Design review of the part built by this model. Coordinates are the model's own, in mm. A direction names the side the tool comes from. Round coordinates to 2 decimals unless told otherwise and drop trailing zeros. Loops run counter-clockwise (first coordinate to the right, second up) from the corner with the lowest first, then second, coordinate; pieces in that order, holes last. Notation, with made-up numbers: M -4.5,-36 L 42.5,-36 A30 cw 42.5,-13 Z; hole C -19.75,53 d7. An arc over 180 degrees is marked long. Use a Markdown table: item, result.
from build123d import *

# Parameters (mm, degrees)
SKETCH1_W                           = 139.991389113
SKETCH1_H                           = 97.393342316
PICOVER_DEPTH                       = 40
PICOVER_DEPTH_BACK                  = 2
SKETCH2_W                           = 96.759944342
SKETCH2_H                           = 90.25941534
OPENINGFORPI_DEPTH                  = 37
SKETCH3_R                           = 23.23056694
HOLETOACCESSSDCARD_DEPTH            = 7.133927
SKETCH4_W                           = 18
SKETCH4_H                           = 97.393342316
CUTAWAYSTHATDEFINESCREWPLATES_DEPTH = 30
BOSS_EXTRUDE1_DEPTH                 = 97.393342
SKETCH6_W                           = 63.672875613
SKETCH6_H                           = 37
HOLEFORPOWERHDMIAUDIO_DEPTH         = 30
SKETCH5_R                           = 2.75
CUT_EXTRUDE5_DEPTH                  = 43
SKETCH7_R                           = 2.75
CUT_EXTRUDE7_DEPTH                  = 30
FILLET1_R                           = 30
FILLET2_R                           = 30


with BuildPart() as part:
    # Sketch1 → PiCover (new body, two sides)
    with BuildSketch(Plane(origin=(0, 0, 0), x_dir=(1, 0, 0), z_dir=(0, 1, 0))) as picover_sk:
        with Locations((69.995694556, 48.696671158)):
            Rectangle(SKETCH1_W, SKETCH1_H)
    extrude(amount=PICOVER_DEPTH)
    extrude(picover_sk.sketch, amount=-PICOVER_DEPTH_BACK)

    # Sketch2 → OpeningForPi (cut)
    with BuildSketch(Plane(origin=(0, 40, 0), x_dir=(1, 0, 0), z_dir=(0, 1, 0))):
        with Locations((70.044375284, 52.263634646)):
            Rectangle(SKETCH2_W, SKETCH2_H)
    extrude(amount=-OPENINGFORPI_DEPTH, mode=Mode.SUBTRACT)

    # Sketch3 → HoleToAccessSDCard (cut)
    with BuildSketch(Plane.XY):
        with Locations((67.175241294, 40)):
            Circle(SKETCH3_R)
    extrude(amount=-HOLETOACCESSSDCARD_DEPTH, mode=Mode.SUBTRACT)

    # Sketch4 → CutAwaysThatDefineScrewPlates (cut)
    with BuildSketch(Plane.XZ.offset(2)):
        with Locations((130.991389113, -48.696671158)):
            Rectangle(SKETCH4_W, SKETCH4_H)
        with Locations((9, -48.696671158)):
            Rectangle(SKETCH4_W, SKETCH4_H)
    extrude(amount=-CUTAWAYSTHATDEFINESCREWPLATES_DEPTH, mode=Mode.SUBTRACT)

    # Sketch11 → Boss-Extrude1 (add)
    with BuildSketch(Plane.XY):
        Polygon((0, 28), (18, 28), (18, -2), align=None)
        Polygon((139.991389113, 28), (121.991389113, 28), (121.991389113, -2), align=None)
    extrude(amount=-BOSS_EXTRUDE1_DEPTH)

    # Sketch6 → HoleForPowerHDMIAudio (cut)
    with BuildSketch(Plane(origin=(21.664403113, 0, 0), x_dir=(0, 0, -1), z_dir=(1, 0, 0))):
        with Locations((44.503037234, 21.5)):
            Rectangle(SKETCH6_W, SKETCH6_H)
    extrude(amount=-HOLEFORPOWERHDMIAUDIO_DEPTH, mode=Mode.SUBTRACT)

    # Sketch5 → Cut-Extrude5 (cut, through all)
    with BuildSketch(Plane(origin=(0, 40, 0), x_dir=(1, 0, 0), z_dir=(0, 1, 0))):
        with Locations((129.624485255, 49.878598174)):
            Circle(SKETCH5_R)
    extrude(amount=-CUT_EXTRUDE5_DEPTH, mode=Mode.SUBTRACT)

    # Sketch7 → Cut-Extrude7 (cut)
    with BuildSketch(Plane(origin=(0, 40, 0), x_dir=(1, 0, 0), z_dir=(0, 1, 0))):
        with Locations((6.934452889, 8.128892452)):
            Circle(SKETCH7_R)
        with Locations((6.934452889, 91.275593332)):
            Circle(SKETCH7_R)
    extrude(amount=-CUT_EXTRUDE7_DEPTH, mode=Mode.SUBTRACT)

    # Fillet1
    fillet1_edges = [part.edges().sort_by_distance(p)[0] for p in [
        (21.664403113, 3, -86.866408678),
    ]]
    fillet(fillet1_edges, radius=FILLET1_R)

    # Fillet2
    fillet2_edges = [part.edges().sort_by_distance(p)[0] for p in [
        (118.424347455, 3, -52.263634646),
    ]]
    fillet(fillet2_edges, radius=FILLET2_R)


solid = part.part
1. The part is to be moulded in two halves that separate along Z. For faces 1 (the face through (126, 40, -49)), 2 (the face through (126.877, 26.996, -50)), 3 (the face through (71, 15, 0)), say which applies: pulls with the +Z half, pulls with the -Z half, needs draft (parallel to the pull), parting line crosses it, or undercut.
Check values:
| item | result |
|---|---|
| face 1 | needs draft |
| face 2 | undercut |
| face 3 | pulls with the +Z half |
2. Take a section at D-D on x = 25.5. Give the boundary of the cut face in (y, z).
Check values:
| item | result |
|---|---|
| outline | M -2,-97.39 L 18.32,-97.39 L 18.32,-76.34 L 3,-76.34 L 3,-7.13 L 40,-7.13 L 40,0 L -2,0 Z |
3. Take a section at C-C on z = -58. Give the boundary of the cut face in (x, y), and give its area (3 significant figures).
Check values:
| item | result |
|---|---|
| outline | M 15,3 L 18,-2 L 121.99,-2 L 139.99,28 L 139.99,40 L 118.42,40 L 118.42,33 A30 cw 88.42,3 Z |
| area | 1,340 mm² |
4. Insertion check: pin 1 (4.5 mm diameter, centred on y = 24.5, z = -9.5, fed in from +X); pin 2 (3 mm diameter, centred on y = 31.5, z = -45, fed in from -X); pin 3 (9 mm diameter, centred on x = 129.62, z = -49.88, fed in from -Y). Each pin has a flat end and moves straight along its axis. Give the tip position at first contact, or say it passes through.
Check values:
| item | result |
|---|---|
| pin 1 | stops at x = 139.24 |
| pin 2 | stops at x = 118.27 |
| pin 3 | stops at y = 3.21 |
5. Take a section at B-B on y = 35. Give the boundary of the cut face in (x, z).
Check values:
| item | result |
|---|---|
| outline | M 0,-97.39 L 21.66,-97.39 L 21.66,-76.34 L 0,-76.34 Z; M 0,-12.67 L 21.66,-12.67 L 21.66,-7.13 L 44.49,-7.13 L 44.49,0 L 0,0 Z; M 89.86,-7.13 L 118.42,-7.13 L 118.42,-97.39 L 139.99,-97.39 L 139.99,0 L 89.86,0 Z; hole C 6.93,-91.28 d5.5; hole C 6.93,-8.13 d5.5; hole C 129.62,-49.88 d5.5 |
6. Machinability: for faces 4 (the face through (30.69, 11.55, -87.01)), 5 (the face through (13, 25, -12.667)), 6 (the face through (22, 40, -5)), which of the approach directions +Z, -Z, +X, -X, +Y, -Y give a long, thin tool a straight path to every point of the face, cutting with its end or side? Answer none if there is none.
Check values:
| item | result |
|---|---|
| face 4 | -Z, +Y |
| face 5 | -X, +Y |
| face 6 | +Z, -Z, +X, -X, +Y |
7. Wall thickness on line 1 along Z through (x, y) = (6.5, 38.5); line 2 along X through (y, z) = (36, -92.5); line 3 along Z through (x, y) = (116, 36): over which ranges is each line inside the solid? List them lowest first. Write a range as from..to.
Check values:
| item | result |
|---|---|
| line 1 | z = -97.39..-93.99, -88.56..-76.34, -12.67..-10.84, -5.41..0 |
| line 2 | x = 0..4.47, 9.4..21.66, 118.42..139.99 |
| line 3 | z = -7.13..0 |
8. Take a section at A-A on y = 20. Give the boundary of the cut face in (x, z).
Check values:
| item | result |
|---|---|
| outline | M 4.8,-97.39 L 24.63,-97.39 L 24.63,-76.34 L 4.8,-76.34 L 4.8,-89.54 A2.75 cw long 4.8,-93.01 Z; M 4.8,-12.67 L 21.66,-12.67 L 21.66,-7.13 L 55.36,-7.13 L 55.36,0 L 4.8,0 L 4.8,-6.39 A2.75 cw long 4.8,-9.86 Z; M 78.99,-7.13 L 115.46,-7.13 L 115.46,-97.39 L 135.19,-97.39 L 135.19,0 L 78.99,0 Z; hole C 129.62,-49.88 d5.5 |
